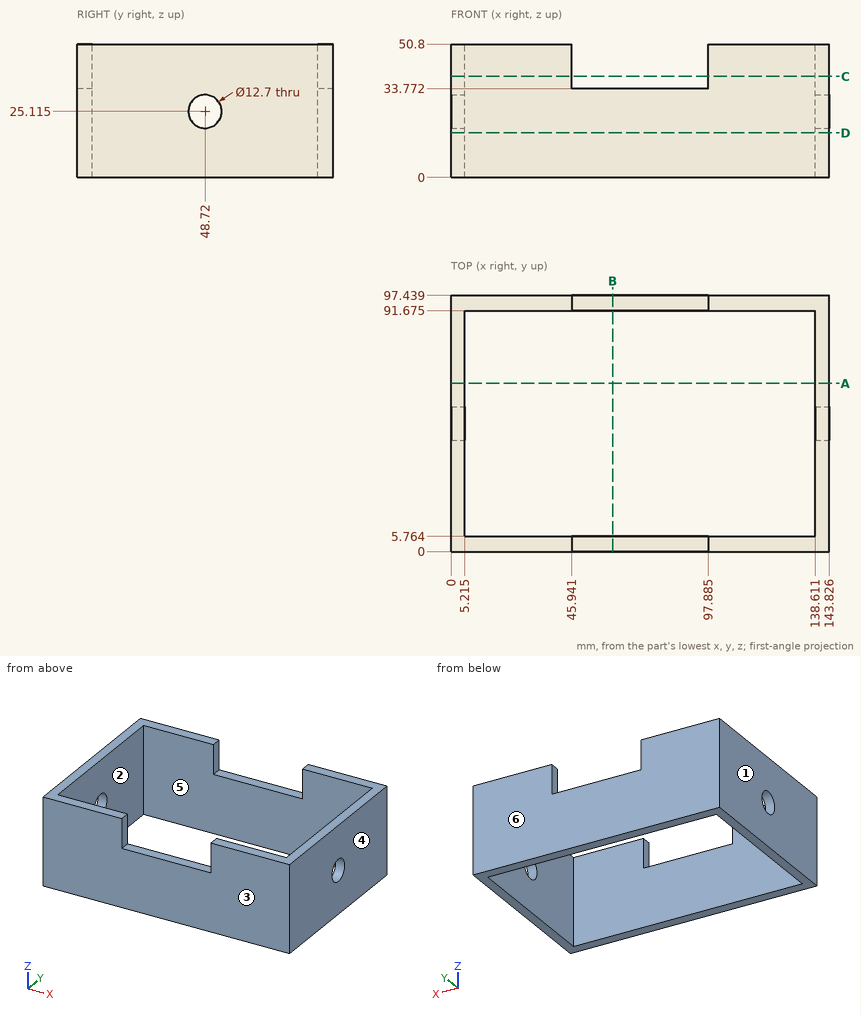
Part print with two shaded views. Sizes in mm from the minimum x, y, z corner. A direction names the side the tool comes from. Coordinates: 2 decimals unless noted, no trailing zeros. Order: outer loops, then holes, each group sorted by start corner. A loop starts at its lowest first (then second) coordinate and runs counter-clockwise, first axis right, second up. Notation, with made-up numbers: (21.5, 85.25) - (63.5, 85.25) arc R25 ccw to (63.5, 120.25) - close; hole circle Ø5 at (1, -36.5). An arc over 180 degrees is marked (long way). Write item = value, one per line. Start each with the question number.
1) Saw through at A-A on y = 64. Write the cut outline in (x, z) (1 decimal).
2) Flat gauge pin, fed straight in: pin 1 Ø3 at (x, y) = (81.5, 4) entering from +Z. Where does the tip first touch, or does it go through?
3) Saw through at D-D on z = 17. Write the cut outline in (x, y) (1 decimal), then the cut area to 3 significant figures.
4) Saw through at B-B on x = 61.5. Write the cut outline in (y, z) (1 decimal), then the cut area to 3 significant figures.
5) Saw through at C-C on z = 38.5. Write the cut outline in (x, y) (1 decimal).
6) 3-axis set-ups, long thin cutter, end or side, ignore diameter. For the marked faces 5 and 6: which of +Z, -Z, +X, -X, +Y, -Y reach the whole face in a straight line?
7) Two-plate mould, pull along X, no slides. Class the marked faces 1, 2, 3 and 4: pulls with the +X half, pulls with the -X half, needs draft (parallel to the pull), parting line crosses it, or undercut.
8) Wall check: line 1 along X through (y, z) = (61, 3) (1 decimal); line 2 along Y through (x, z) = (115, 48) (1 decimal); line 3 along Z through (x, y) = (54, 93.5). Give the ranges that are in metal, low to high. Write a range as from..to.
From the geometry:
q1.outline = (0, 0) - (5.2, 0) - (5.2, 50.8) - (0, 50.8) - close; (138.6, 0) - (143.8, 0) - (143.8, 50.8) - (138.6, 50.8) - close
q2.pin_1 = 33.77
q3.outline = (0, 0) - (143.8, 0) - (143.8, 97.4) - (0, 97.4) - close; hole (5.2, 5.8) - (138.6, 5.8) - (138.6, 91.7) - (5.2, 91.7) - close
q3.area = 2,550 mm^2
q4.outline = (0, 0) - (5.8, 0) - (5.8, 33.8) - (0, 33.8) - close; (91.7, 0) - (97.4, 0) - (97.4, 33.8) - (91.7, 33.8) - close
q4.area = 389 mm^2
q5.outline = (0, 0) - (45.9, 0) - (45.9, 5.8) - (5.2, 5.8) - (5.2, 91.7) - (45.9, 91.7) - (45.9, 97.4) - (0, 97.4) - close; (97.9, 0) - (143.8, 0) - (143.8, 97.4) - (97.9, 97.4) - (97.9, 91.7) - (138.6, 91.7) - (138.6, 5.8) - (97.9, 5.8) - close
q6.face_5 = +Z, -Z
q6.face_6 = +Z, -Z, +X, -X, +Y
q7.face_1 = pulls with the -X half
q7.face_2 = undercut
q7.face_3 = needs draft
q7.face_4 = pulls with the +X half
q8.line_1 = 0..5.2, 138.6..143.8
q8.line_2 = 0..5.8, 91.7..97.4
q8.line_3 = 0..33.77
